Geometry check sheet. Reference: the model listing, model coordinates, mm. A direction names the side the tool comes from. Coordinates: 2 decimals unless noted, no trailing zeros. Write each loop counter-clockwise with the first axis right and the second up, starting at its lowest first coordinate (ties: lowest second). Pieces come first, ordered by that corner, then holes. Notation, with made-up numbers: (80, -32) -> (100, -32) arc R36 ccw to (100, 4) -> close; hole circle Ø3 at (58.25, -32). An arc over 180 degrees is marked (long way). Put each result on its own line as item: value. Start each with the question number.
from build123d import *

# Parameters (mm, degrees)
SKETCH_1_W          = 34
SKETCH_1_H          = 26.5
EXTRUDE_1_DEPTH     = 1.7
SKETCH_2_W          = 16
SKETCH_2_H          = 16
EXTRUDE_2_DEPTH     = 12
SKETCH_3_W          = 10
SKETCH_3_H          = 6.5
EXTRUDE_3_DEPTH     = 3
SKETCH_4_W          = 6
SKETCH_4_H          = 6
EXTRUDE_4_DEPTH     = 2.5
SKETCH_5_R          = 1.553190153
EXTRUDE_5_DEPTH     = 0.5
SKETCH_6_W          = 10
SKETCH_6_H          = 3.5
SKETCH_6_W_2        = 3.5
SKETCH_6_H_2        = 10
EXTRUDE_6_DEPTH     = 12
CHAMFER_1_SIZE      = 1
SKETCH_7_R          = 5.5
CUT_EXTRUDE_1_DEPTH = 5
SKETCH_8_W          = 4
SKETCH_8_H          = 3
EXTRUDE_7_DEPTH     = 12.5
CHAMFER_2_SIZE      = 0.5
SKETCH_9_R          = 1.5
CUT_EXTRUDE_2_DEPTH = 30.065658431
SKETCH_10_W         = 1
SKETCH_10_H         = 1
CUT_EXTRUDE_3_DEPTH = 30.065658431


with BuildPart() as part:
    # Эскиз1 → Бобышка-Вытянуть1 (new body)
    with BuildSketch(Plane.XY):
        Rectangle(SKETCH_1_W, SKETCH_1_H)
    extrude(amount=EXTRUDE_1_DEPTH)

    # Эскиз2 → Бобышка-Вытянуть2 (add)
    with BuildSketch(Plane.XY.offset(1.7)):
        with Locations((0, 1.25)):
            Rectangle(SKETCH_2_W, SKETCH_2_H)
    extrude(amount=EXTRUDE_2_DEPTH)

    # Эскиз3 → Бобышка-Вытянуть3 (add)
    with BuildSketch(Plane.XY.offset(1.7)):
        with Locations((0, -10)):
            Rectangle(SKETCH_3_W, SKETCH_3_H)
    extrude(amount=EXTRUDE_3_DEPTH)

    # Эскиз4 → Бобышка-Вытянуть4 (add)
    with BuildSketch(Plane.XY.offset(4.7)):
        with Locations((0, -10)):
            Rectangle(SKETCH_4_W, SKETCH_4_H)
    extrude(amount=EXTRUDE_4_DEPTH)

    # Эскиз5 → Бобышка-Вытянуть5 (add)
    with BuildSketch(Plane.XY.offset(7.2)):
        with Locations((0, -10)):
            Circle(SKETCH_5_R)
    extrude(amount=EXTRUDE_5_DEPTH)

    # Эскиз6 → Бобышка-Вытянуть6 (add)
    with BuildSketch(Plane.XY.offset(1.7)):
        with Locations((0, 11)):
            Rectangle(SKETCH_6_W, SKETCH_6_H)
        with Locations((9.75, 1.25)):
            Rectangle(SKETCH_6_W_2, SKETCH_6_H_2)
    extrude(amount=EXTRUDE_6_DEPTH)

    # Фаска1
    chamfer_1_edges = [part.edges().sort_by_distance(p)[0] for p in [
        (5, 12.75, 7.7),
        (-5, 12.75, 7.7),
        (11.5, -3.75, 7.7),
        (11.5, 6.25, 7.7),
    ]]
    chamfer(chamfer_1_edges, length=CHAMFER_1_SIZE)

    # Эскиз7 → Вырез-Вытянуть1 (cut)
    with BuildSketch(Plane.XY.offset(13.7)):
        with Locations((0, 1.25)):
            Circle(SKETCH_7_R)
    extrude(amount=-CUT_EXTRUDE_1_DEPTH, mode=Mode.SUBTRACT)

    # Эскиз8 → Бобышка-Вытянуть7 (add)
    with BuildSketch(Plane.XY.offset(8.7)):
        with Locations((0, 1.25)):
            Rectangle(SKETCH_8_W, SKETCH_8_H)
    extrude(amount=EXTRUDE_7_DEPTH)

    # Фаска2
    chamfer_2_edges = [part.edges().sort_by_distance(p)[0] for p in [
        (2, 1.25, 8.7),
        (2, -0.25, 14.95),
        (0, 2.75, 8.7),
        (2, 2.75, 14.95),
        (-2, 1.25, 8.7),
        (-2, 2.75, 14.95),
        (0, -0.25, 8.7),
        (-2, -0.25, 14.95),
        (2, 1.25, 21.2),
        (0, 2.75, 21.2),
        (-2, 1.25, 21.2),
        (0, -0.25, 21.2),
    ]]
    chamfer(chamfer_2_edges, length=CHAMFER_2_SIZE)

    # Эскиз9 → Вырез-Вытянуть2 (cut, through all)
    with BuildSketch(Plane.XY.offset(1.7)):
        with Locations((14, 10.25)):
            Circle(SKETCH_9_R)
        with Locations((14, -10.25)):
            Circle(SKETCH_9_R)
        with Locations((-12, 10.25)):
            Circle(SKETCH_9_R)
        with Locations((-12, -10.25)):
            Circle(SKETCH_9_R)
    extrude(amount=-CUT_EXTRUDE_2_DEPTH, mode=Mode.SUBTRACT)

    # Эскиз10 → Вырез-Вытянуть3 (cut, through all)
    with BuildSketch(Plane.XY.offset(1.7)):
        with Locations((-14.5, 2.364432177)):
            Rectangle(SKETCH_10_W, SKETCH_10_H)
        with Locations((-14.5, 4.904432177)):
            Rectangle(SKETCH_10_W, SKETCH_10_H)
        with Locations((-14.5, -0.175567823)):
            Rectangle(SKETCH_10_W, SKETCH_10_H)
        with Locations((-14.5, -2.715567823)):
            Rectangle(SKETCH_10_W, SKETCH_10_H)
        with Locations((-14.5, -5.255567823)):
            Rectangle(SKETCH_10_W, SKETCH_10_H)
    extrude(amount=-CUT_EXTRUDE_3_DEPTH, mode=Mode.SUBTRACT)


solid = part.part
Item 1: Access from +Z, -Z, +X, -X, +Y, -Y to the whole of each face (thin tool, end or side, straight path). Record for faces 1 (the flat face through (-14.5, 0.324, 0.9)), 2 (the flat face through (0, -13, 6)), 3 (the flat face through (2, 1, 15)).
Item 2: Go/stop test with flat-tipped pins: P1, Ø1.5, axis at y = -7, z = 14, coming from the -X side; P2, Ø3, axis at x = -0.5, z = 14.5, coming from the +Y side; P3, Ø4, axis at x = 6.5, z = 7.5, coming from the +Y side; P4, Ø6, axis at y = -5.5, z = 18.5, coming from the -X side. Record where each tip stops, or that it passes through.
Item 3: Scan lines: line 1 along Y through (x, z) = (14, 0.75); line 2 along Y through (x, z) = (0.5, 12.75); line 3 along Z through (x, y) = (4.5, -10). Record each from-to range of solid material in increasing order. Write a range as [from, to].
Item 4: Section check A-A, the plane x = 14. Enter the section's corners in (y, z).
Item 5: Section check B-B, the plane x = -14.5. Enter the section's corners in (y, z).
Item 6: Section check D-D, the plane y = 7.5. Enter the section's corners in (x, z), and give its area (3 significant figures).
Item 7: Section check C-C, the plane z = 2.25. Enter the section's corners in (x, y).
Item 8: Mould release check, pull along X, two halves, no side actions. Record for faces 4 (the flat face through (10.99, 5.76, 7.62)), 5 (the flat face through (-1.91, -0.14, 8.9)), 6 (the flat face through (-8, 1, 8)): released by +X, released by -X, zero draft, split by the parting line, or undercut.
From the geometry:
1. face 1: +Z, -Z
1. face 2: +Z, +X, -X, -Y
1. face 3: +Z
2. P1: x = -8
2. P2: y = 12.75
2. P3: y = 12.25
2. P4: through
3. line 1: [-13.25, -11.75], [-8.75, 8.75], [11.75, 13.25]
3. line 2: [-6.75, -4.23], [-0.25, 2.75], [6.73, 12.75]
3. line 3: [0, 4.7]
4. outline: (-13.25, 0) -> (-11.75, 0) -> (-11.75, 1.7) -> (-13.25, 1.7) -> close; (-8.75, 0) -> (8.75, 0) -> (8.75, 1.7) -> (-8.75, 1.7) -> close; (11.75, 0) -> (13.25, 0) -> (13.25, 1.7) -> (11.75, 1.7) -> close
5. outline: (-13.25, 0) -> (-5.76, 0) -> (-5.76, 1.7) -> (-13.25, 1.7) -> close; (-4.76, 0) -> (-3.22, 0) -> (-3.22, 1.7) -> (-4.76, 1.7) -> close; (-2.22, 0) -> (-0.68, 0) -> (-0.68, 1.7) -> (-2.22, 1.7) -> close; (0.32, 0) -> (1.86, 0) -> (1.86, 1.7) -> (0.32, 1.7) -> close; (2.86, 0) -> (4.4, 0) -> (4.4, 1.7) -> (2.86, 1.7) -> close; (5.4, 0) -> (13.25, 0) -> (13.25, 1.7) -> (5.4, 1.7) -> close
6. outline: (-17, 0) -> (17, 0) -> (17, 1.7) -> (8, 1.7) -> (8, 13.7) -> (-8, 13.7) -> (-8, 1.7) -> (-17, 1.7) -> close
6. area: 250 mm²
7. outline: (-8, -6.75) -> (-5, -6.75) -> (-5, -13.25) -> (5, -13.25) -> (5, -6.75) -> (8, -6.75) -> (8, -3.75) -> (10.5, -3.75) -> (11.5, -2.75) -> (11.5, 5.25) -> (10.5, 6.25) -> (8, 6.25) -> (8, 9.25) -> (5, 9.25) -> (5, 11.75) -> (4, 12.75) -> (-4, 12.75) -> (-5, 11.75) -> (-5, 9.25) -> (-8, 9.25) -> close
8. face 4: released by +X
8. face 5: undercut
8. face 6: released by -X
